Could you check a few things on this model? Use its own coordinates, in mm. A direction names the side the tool comes from. Round coordinates to 2 decimals unless told otherwise and drop trailing zeros. Loops run counter-clockwise (first coordinate to the right, second up) from the corner with the lowest first, then second, coordinate; pieces in that order, holes last.
from build123d import *

# Parameters (mm, degrees)
SKETCH1_W           = 76.2
SKETCH1_H           = 25.4
SKETCH1_W_2         = 69.85
SKETCH1_H_2         = 19.05
EXTRUDE_THIN1_DEPTH = 533.4
SKETCH3_R           = 24.97201
CUT_EXTRUDE2_DEPTH  = 26.4
SKETCH4_R           = 3.175
CUT_EXTRUDE3_DEPTH  = 77.2


with BuildPart() as part:
    # Sketch1 → Extrude-Thin1 (new body)
    with BuildSketch(Plane.XY):
        Rectangle(SKETCH1_W, SKETCH1_H)
        Rectangle(SKETCH1_W_2, SKETCH1_H_2, mode=Mode.SUBTRACT)
    extrude(amount=EXTRUDE_THIN1_DEPTH)

    # Sketch3 → Cut-Extrude2 (cut, through all)
    with BuildSketch(Plane(origin=(0, 12.7, 0), x_dir=(1, 0, 0), z_dir=(0, 1, 0))):
        with Locations((0, -34.49701)):
            Circle(SKETCH3_R)
        with Locations((0, -498.90299)):
            Circle(SKETCH3_R)
    extrude(amount=-CUT_EXTRUDE2_DEPTH, mode=Mode.SUBTRACT)

    # Sketch4 → Cut-Extrude3 (cut, through all)
    with BuildSketch(Plane(origin=(38.1, 0, 0), x_dir=(0, 0, -1), z_dir=(1, 0, 0))):
        with Locations((-34.49701, 0)):
            Circle(SKETCH4_R)
        with Locations((-498.90299, 0)):
            Circle(SKETCH4_R)
    extrude(amount=-CUT_EXTRUDE3_DEPTH, mode=Mode.SUBTRACT)


solid = part.part
Item 1: If we section it at B-B, the plane x = -16: Please give me the cut outline in (y, z) (3 decimals), then the cut area to 3 significant figures.
Results list:
outline: (-12.7, 0) - (-9.525, 0) - (-9.525, 15.324) - (-12.7, 15.324) - close; (-12.7, 53.67) - (-9.525, 53.67) - (-9.525, 479.73) - (-12.7, 479.73) - close; (-12.7, 518.076) - (-9.525, 518.076) - (-9.525, 533.4) - (-12.7, 533.4) - close; (9.525, 0) - (12.7, 0) - (12.7, 15.324) - (9.525, 15.324) - close; (9.525, 53.67) - (12.7, 53.67) - (12.7, 479.73) - (9.525, 479.73) - close; (9.525, 518.076) - (12.7, 518.076) - (12.7, 533.4) - (9.525, 533.4) - close
area: 2,900 mm2
Item 2: If I drill on line 1 along Y through (x, z) = (-20.5, 184.5) (3 decimals); line 2 along Z through (x, y) = (0, -10.4) (3 decimals); line 3 along X through (y, z) = (6.75, 121) (3 decimals), over which ranges is the centre line in solid material (lowest first)?
Results list:
line 1: y = -12.7 to -9.525, 9.525 to 12.7
line 2: z = 0 to 9.525, 59.469 to 473.931, 523.875 to 533.4
line 3: x = -38.1 to -34.925, 34.925 to 38.1
Item 3: Will this pin go through, and if not, where does the flat tip stop? pin 1 (5.5 mm diameter, centred on y = 0, z = 498.9, fed in from +X).
Results list:
pin 1: passes through
Item 4: For faces 1 (the flat face through (0, 9.525, 263)), 2 (the cylindrical face through (-3.251, 11.135, 9.738)), which set-ups out of +Z, -Z, +X, -X, +Y, -Y let a thin tool reach every point of the face, with its end or its side?
Results list:
face 1: +Z, -Z
face 2: +Y, -Y
Item 5: We'd pull the mould along X, two halves only. Please class faces 3 (the flat face through (0, -9.525, 263)), 4 (the flat face through (38.1, 0, 263)), 5 (the flat face through (-38.1, 0, 263)): released by +X, released by -X, zero draft, split by the parting line, or undercut.
Results list:
face 3: undercut
face 4: released by +X
face 5: released by -X
Item 6: If we section it at A-A, the plane z = 427: Please give me the cut outline in (x, y) (3 decimals).
Results list:
outline: (-38.1, -12.7) - (38.1, -12.7) - (38.1, 12.7) - (-38.1, 12.7) - close; hole (-34.925, -9.525) - (34.925, -9.525) - (34.925, 9.525) - (-34.925, 9.525) - close
Item 7: If we section it at C-C, the plane z = 44: Please give me the cut outline in (x, y) (3 decimals).
Results list:
outline: (-38.1, -12.7) - (-23.093, -12.7) - (-23.093, -9.525) - (-34.925, -9.525) - (-34.925, 9.525) - (-23.093, 9.525) - (-23.093, 12.7) - (-38.1, 12.7) - close; (23.093, -12.7) - (38.1, -12.7) - (38.1, 12.7) - (23.093, 12.7) - (23.093, 9.525) - (34.925, 9.525) - (34.925, -9.525) - (23.093, -9.525) - close
